Can you work these out from the drawing? Everything is in mm from the part's minimum corner. A direction names the side the tool comes from. Round coordinates to 2 decimals unless told otherwise and drop trailing zeros. Loops run counter-clockwise (first coordinate to the right, second up) from the corner with the lowest first, then second, coordinate; pieces in that order, holes last. Notation, with made-up numbers: M -20,30.5 L 16,30.5 A13 cw 16,45.5 Z; hole C 18,-18 d6. An arc over 180 degrees is marked long. One line per question, with ' | ' between items. Start each with the question number.
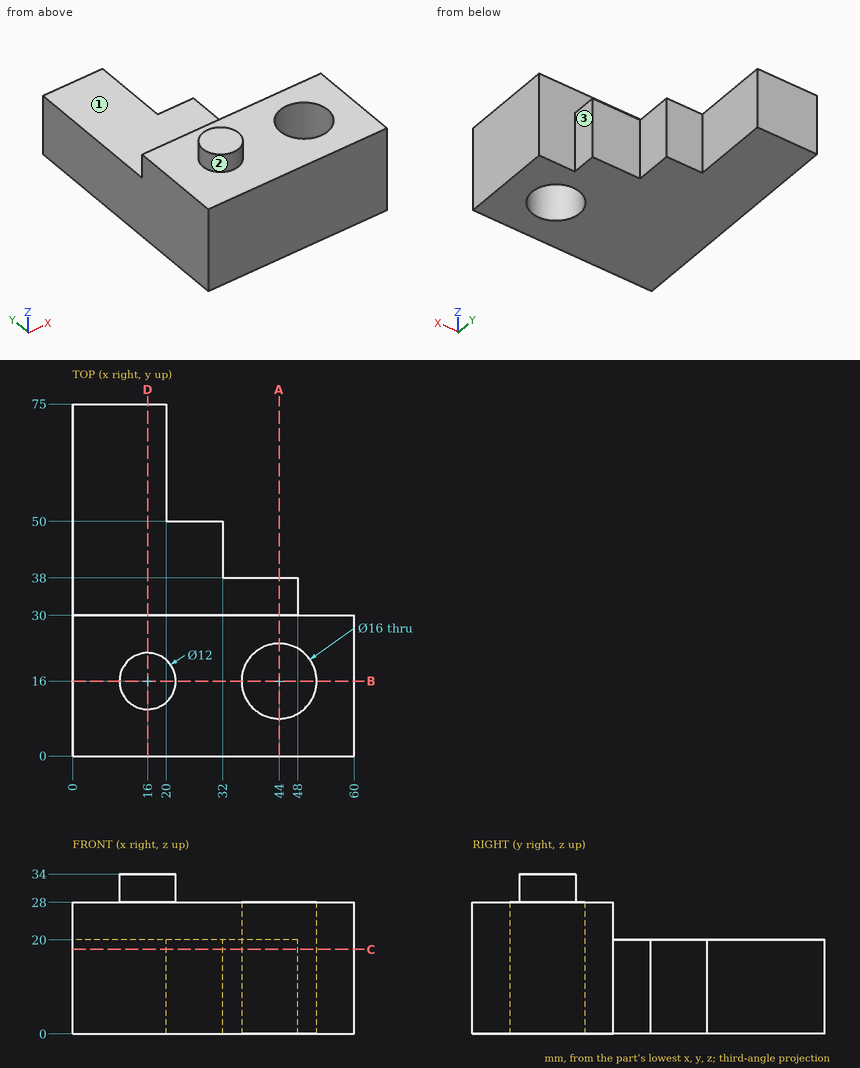
1) I'm going to push flat-ended pins straight in: pin 1 Ø17.5 at (x, z) = (42, 14.5) entering from +Y; pin 2 Ø10 at (x, y) = (25, 27.5) entering from +Z; pin 3 Ø6 at (y, z) = (43.5, 8) entering from +X; pin 4 Ø3 at (y, z) = (11.5, 8.5) entering from -X. Where does each tip first touch, or does it pass through?
2) Please list where these lines run through material, in increasing order: L1, parallel to Y at x = 44, z = 17.5; L2, parallel to Z at x = 22, y = 32; L3, parallel to Z at x = 28, y = 25. Write a range as from..to.
3) Imagine slicing it at C-C (z = 18). Write out the boundary of the cut face in (x, y).
4) Imagine slicing it at B-B (y = 16). Write out the boundary of the cut face in (x, z), then the cut area to 3 significant figures.
5) Imagine slicing it at D-D (x = 16). Write out the boundary of the cut face in (y, z), then the cut area to 3 significant figures.
6) Imagine slicing it at A-A (x = 44). Write out the boundary of the cut face in (y, z), then the cut area to 3 significant figures.
7) For the marked faces 1, 2 and 3, which set-ups out of +Z, -Z, +X, -X, +Y, -Y let a thin tool reach every point of the face, with its end or its side?
Results are:
1) pin 1: y = 38 | pin 2: z = 28 | pin 3: x = 32 | pin 4: x = 0
2) L1: 0..8, 24..38 | L2: 0..20 | L3: 0..28
3) outline: M 0,0 L 60,0 L 60,30 L 48,30 L 48,38 L 32,38 L 32,50 L 20,50 L 20,75 L 0,75 Z; hole C 44,16 d16
4) outline: M 0,0 L 36,0 L 36,28 L 22,28 L 22,34 L 10,34 L 10,28 L 0,28 Z; M 52,0 L 60,0 L 60,28 L 52,28 Z | area: 1,300 mm²
5) outline: M 0,0 L 75,0 L 75,20 L 30,20 L 30,28 L 22,28 L 22,34 L 10,34 L 10,28 L 0,28 Z | area: 1,810 mm²
6) outline: M 0,0 L 8,0 L 8,28 L 0,28 Z; M 24,0 L 38,0 L 38,20 L 30,20 L 30,28 L 24,28 Z | area: 552 mm²
7) face 1: +Z, +X, -X, +Y | face 2: +Z | face 3: +Z, -Z, +X, +Y
